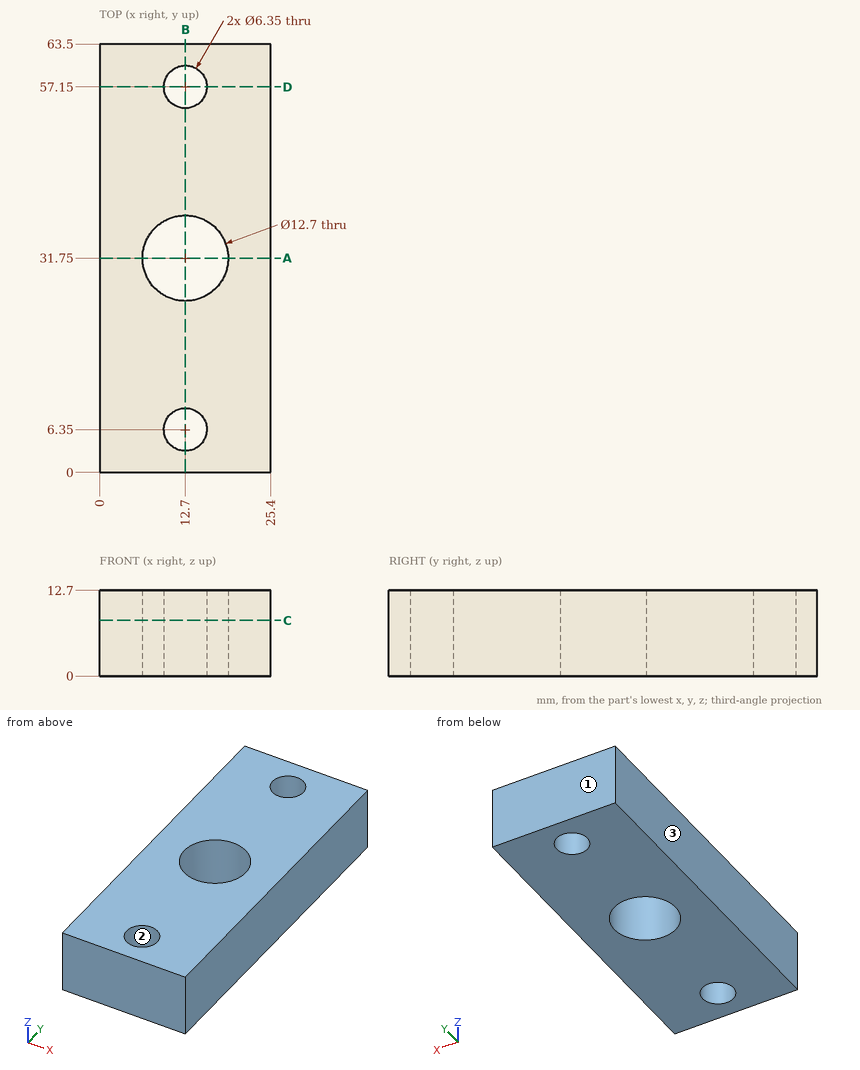
Geometry: see drawing. Coordinates: mm, zero at the bounding-box minimum. Coordinates: 2 decimals unless noted, no trailing zeros. Write each loop counter-clockwise with the first axis right and the second up, starting at its lowest first coordinate (ties: lowest second). Pieces come first, ordered by that corner, then holes. Notation, with made-up numbers: (-30.5, 79) - (11.5, 79) arc R34 ccw to (11.5, 116) - close; hole circle Ø7 at (65, -29.5). An arc over 180 degrees is marked (long way). Put each result on its own line as item: value. Start each with the question number.
1) Ray query, L1, parallel to Y at x = 12.7, z = 4.5 (3 decimals); L2, parallel to X at y = 6.35, z = 5 (3 decimals); L3, parallel to X at y = 31.75, z = 9. Return the intervals inside material, ascending.
2) Contact query for a flat-ended pin moving along its axis: pin 1 (6 mm diameter, centred on x = 19.5, z = 4, fed in from -Y). Output: stop coordinate, or through.
3) Cut plane C-C (z = 8.25). Return the cut outline in (x, y) (3 decimals), plus the area to 3 significant figures.
4) Cut plane B-B (x = 12.7). Return the cut outline in (y, z) (3 decimals).
5) Cut plane A-A (y = 31.75). Return the cut outline in (x, z), plus the area to 3 significant figures.
6) Mould query, pull axis X, two halves, no side actions, for the marked faces 1, 2 and 3. Classes: pulls with the +X half, pulls with the -X half, needs draft (parallel to the pull), parting line crosses it, or undercut.
7) Cut plane D-D (y = 57.15). Return the cut outline in (x, z) (3 decimals), plus the area to 3 significant figures.
Resolved:
1. L1: y = 0 to 3.175, 9.525 to 25.4, 38.1 to 53.975, 60.325 to 63.5
1. L2: x = 0 to 9.525, 15.875 to 25.4
1. L3: x = 0 to 6.35, 19.05 to 25.4
2. pin 1: stops at y = 0
3. outline: (0, 0) - (25.4, 0) - (25.4, 63.5) - (0, 63.5) - close; hole circle Ø12.7 at (12.7, 31.75); hole circle Ø6.35 at (12.7, 6.35); hole circle Ø6.35 at (12.7, 57.15)
3. area: 1,420 mm2
4. outline: (0, 0) - (3.175, 0) - (3.175, 12.7) - (0, 12.7) - close; (9.525, 0) - (25.4, 0) - (25.4, 12.7) - (9.525, 12.7) - close; (38.1, 0) - (53.975, 0) - (53.975, 12.7) - (38.1, 12.7) - close; (60.325, 0) - (63.5, 0) - (63.5, 12.7) - (60.325, 12.7) - close
5. outline: (0, 0) - (6.35, 0) - (6.35, 12.7) - (0, 12.7) - close; (19.05, 0) - (25.4, 0) - (25.4, 12.7) - (19.05, 12.7) - close
5. area: 161 mm2
6. face 1: needs draft
6. face 2: undercut
6. face 3: pulls with the -X half
7. outline: (0, 0) - (9.525, 0) - (9.525, 12.7) - (0, 12.7) - close; (15.875, 0) - (25.4, 0) - (25.4, 12.7) - (15.875, 12.7) - close
7. area: 242 mm2
